Source: three-view drawing plus pictorial views. Frame: mm from the lowest corner of the part. A direction names the side the tool comes from. Round coordinates to 2 decimals unless told otherwise and drop trailing zeros. Order: outer loops, then holes, each group sorted by start corner. A loop starts at its lowest first (then second) coordinate and runs counter-clockwise, first axis right, second up. Notation, with made-up numbers: (82, -19.75) -> (98, -19.75) arc R20 ccw to (98, 0.25) -> close; hole circle Ø1 at (-33, -26.5). An arc over 180 degrees is marked (long way). Use a Markdown table: item, result.
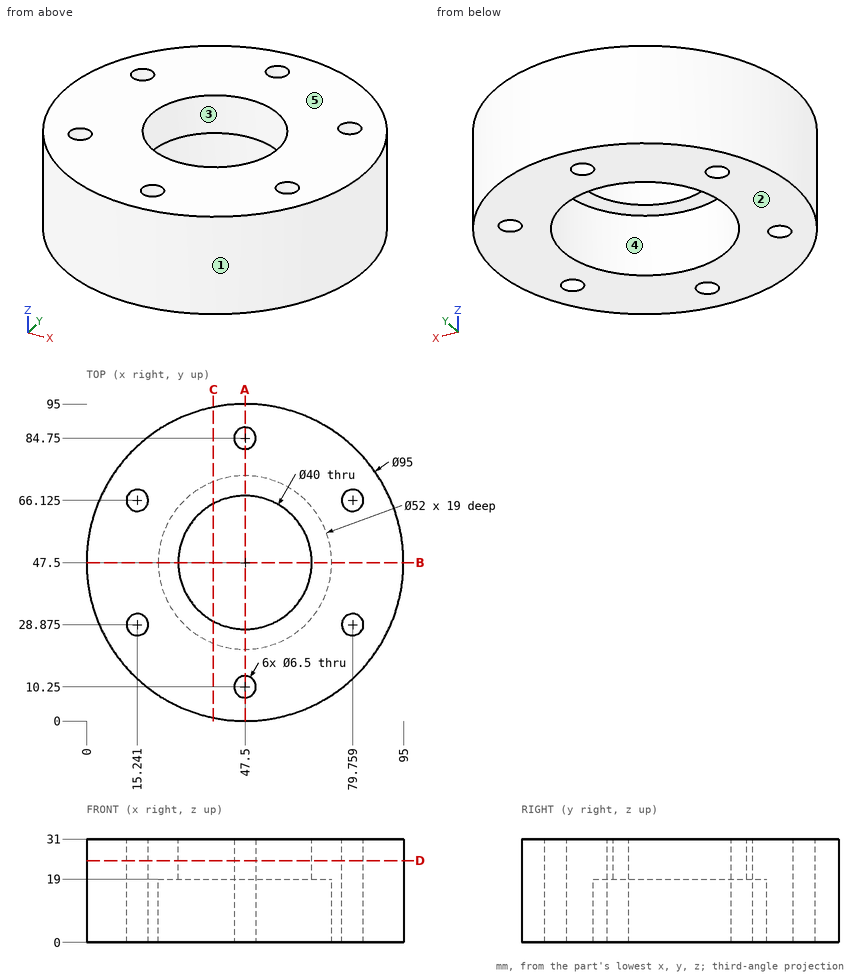
1) Cut plane D-D on z = 24.5. Count the separate pieces of the cut face and the enclosed holes in it, and give its area (3 significant figures).
Results found:
| item | result |
|---|---|
| separate pieces | 1 |
| enclosed holes | 7 |
| area | 5,630 mm² |
2) Line query: L1, parallel to Y at x = 47.5, z = 9; L2, parallel to Y at x = 12.5, z = 16.5 (1 decimal); L3, parallel to Y at x = 47, z = 24. Output: solid intervals per line, ascending. Write a range as [from, to].
Results found:
| item | result |
|---|---|
| L1 | y = [0, 7], [13.5, 21.5], [73.5, 81.5], [88, 95] |
| L2 | y = [15.4, 27.1], [30.6, 64.4], [67.9, 79.6] |
| L3 | y = [0, 7.04], [13.46, 27.51], [67.49, 81.54], [87.96, 95] |
3) Cut plane B-B on y = 47.5. Return loops of the section in (x, z).
Results found:
| item | result |
|---|---|
| outline | (0, 0) -> (21.5, 0) -> (21.5, 19) -> (27.5, 19) -> (27.5, 31) -> (0, 31) -> close; (67.5, 19) -> (73.5, 19) -> (73.5, 0) -> (95, 0) -> (95, 31) -> (67.5, 31) -> close |
4) Cut plane C-C on x = 38. Return loops of the section in (y, z).
Results found:
| item | result |
|---|---|
| outline | (0.96, 0) -> (23.3, 0) -> (23.3, 19) -> (29.9, 19) -> (29.9, 31) -> (0.96, 31) -> close; (65.1, 19) -> (71.7, 19) -> (71.7, 0) -> (94.04, 0) -> (94.04, 31) -> (65.1, 31) -> close |
5) Pull-direction query (X, two-part tool) for the marked faces 1, 2 and 3; classes: +X half, -X half, draft (parallel to the pull), parting line (faces both ways), or undercut.
Results found:
| item | result |
|---|---|
| face 1 | parting line |
| face 2 | draft |
| face 3 | undercut |
6) Pin query (flat end, axial travel): pin 1 Ø4 at (x, z) = (30, 9.5) entering from +Y; pin 2 Ø1.5 at (y, z) = (22.5, 22.5) entering from -X; pin 3 Ø8 at (y, z) = (38, 12) entering from +X; pin 4 Ø8.5 at (x, y) = (79.76, 66.12) entering from +Z. Return the tip coordinate at first contact, or that it passes through.
Results found:
| item | result |
|---|---|
| pin 1 | stops at y = 92.4 |
| pin 2 | stops at x = 6.66 |
| pin 3 | stops at x = 94.68 |
| pin 4 | stops at z = 31 |
7) Set-up query: the marked faces 4 and 5. Return all of +Z, -Z, +X, -X, +Y, -Y with unobstructed straight access to the full face (end or side cutting, diameter ignored); none if empty.
Results found:
| item | result |
|---|---|
| face 4 | -Z |
| face 5 | +Z, +X, -X, +Y, -Y |
8) Cut plane A-A on x = 47.5. Return loops of the section in (y, z).
Results found:
| item | result |
|---|---|
| outline | (0, 0) -> (7, 0) -> (7, 31) -> (0, 31) -> close; (13.5, 0) -> (21.5, 0) -> (21.5, 19) -> (27.5, 19) -> (27.5, 31) -> (13.5, 31) -> close; (67.5, 19) -> (73.5, 19) -> (73.5, 0) -> (81.5, 0) -> (81.5, 31) -> (67.5, 31) -> close; (88, 0) -> (95, 0) -> (95, 31) -> (88, 31) -> close |
